CAD build for the part. Positions are in the model's coordinates, mm. A direction names the side the tool comes from. Coordinates: 2 decimals unless noted, no trailing zeros. Loops run counter-clockwise (first coordinate to the right, second up) from the corner with the lowest first, then second, coordinate; pieces in that order, holes last. Notation, with made-up numbers: (-4, 8) - (36, 8) arc R24 ccw to (36, 28) - close; hole circle Ø8 at (-11.75, 44). An arc over 180 degrees is marked (long way). Put each result on its own line as item: value.
```python
from build123d import *

# Parameters (mm, degrees)
SKETCH_1_W          = 15
SKETCH_1_H          = 15
SKETCH_1_W_2        = 13
SKETCH_1_H_2        = 13
EXTRUDE_1_DEPTH     = 460
SKETCH_2_R          = 1.45
CUT_EXTRUDE_1_DEPTH = 461.305605006
SKETCH_3_R          = 1.45
CUT_EXTRUDE_2_DEPTH = 461.305605006


with BuildPart() as part:
    # 草图1 → 拉伸-薄壁1 (new body)
    with BuildSketch(Plane(origin=(0, 0, 0), x_dir=(1, 0, 0), z_dir=(0, 1, 0))):
        Rectangle(SKETCH_1_W, SKETCH_1_H)
        Rectangle(SKETCH_1_W_2, SKETCH_1_H_2, mode=Mode.SUBTRACT)
    extrude(amount=EXTRUDE_1_DEPTH)

    # 草图2 → 切除-拉伸1 (cut, through all)
    with BuildSketch(Plane.XY.offset(7.5)):
        with Locations((0, 7.5)):
            Circle(SKETCH_2_R)
        with Locations((0, 27.5)):
            Circle(SKETCH_2_R)
        with Locations(Location((0, 432.5, 0), (0, 0, 180))):
            Circle(SKETCH_2_R)
        with Locations(Location((0, 452.5, 0), (0, 0, 180))):
            Circle(SKETCH_2_R)
        with Locations((0, 140)):
            Circle(SKETCH_2_R)
        with Locations((0, 160)):
            Circle(SKETCH_2_R)
        with Locations((0, 120)):
            Circle(SKETCH_2_R)
        with Locations(Location((0, 340, 0), (0, 0, 180))):
            Circle(SKETCH_2_R)
        with Locations(Location((0, 300, 0), (0, 0, 180))):
            Circle(SKETCH_2_R)
        with Locations(Location((0, 320, 0), (0, 0, 180))):
            Circle(SKETCH_2_R)
        with Locations((0, 230)):
            Circle(SKETCH_2_R)
        with Locations((0, 255)):
            Circle(SKETCH_2_R)
        with Locations((0, 205)):
            Circle(SKETCH_2_R)
        with Locations((0, 47.5)):
            Circle(SKETCH_2_R)
        with Locations((0, 67.5)):
            Circle(SKETCH_2_R)
        with Locations((0, 87.5)):
            Circle(SKETCH_2_R)
        with Locations((0, 360)):
            Circle(SKETCH_2_R)
        with Locations((0, 380)):
            Circle(SKETCH_2_R)
        with Locations((0, 400)):
            Circle(SKETCH_2_R)
    extrude(amount=-CUT_EXTRUDE_1_DEPTH, mode=Mode.SUBTRACT)

    # 草图3 → 切除-拉伸2 (cut, through all)
    with BuildSketch(Plane(origin=(7.5, 0, 0), x_dir=(0, 0, -1), z_dir=(1, 0, 0))):
        with Locations((0, 152.5)):
            Circle(SKETCH_3_R)
        with Locations((0, 172.5)):
            Circle(SKETCH_3_R)
        with Locations((0, 287.5)):
            Circle(SKETCH_3_R)
        with Locations((0, 307.5)):
            Circle(SKETCH_3_R)
        with Locations((0, 192.5)):
            Circle(SKETCH_3_R)
        with Locations((0, 267.5)):
            Circle(SKETCH_3_R)
    extrude(amount=-CUT_EXTRUDE_2_DEPTH, mode=Mode.SUBTRACT)


solid = part.part
```
Q1. Slice it at B-B, the plane y = 59.5. Give the cut face in (x, z), then the cut area to 3 significant figures.
Determined:
outline: (-7.5, -7.5) - (7.5, -7.5) - (7.5, 7.5) - (-7.5, 7.5) - close; hole (-6.5, -6.5) - (6.5, -6.5) - (6.5, 6.5) - (-6.5, 6.5) - close
area: 56.0 mm2
Q2. Slice it at A-A, the plane x = 4.25. Give the cut face in (y, z).
Determined:
outline: (0, -7.5) - (460, -7.5) - (460, -6.5) - (0, -6.5) - close; (0, 6.5) - (460, 6.5) - (460, 7.5) - (0, 7.5) - close
Q3. Mould opens along Z. For faces 1 (the flat face through (0, 227, -7.5)), 2 (the flat face through (-7.5, 227, 0)), 3 (the flat face through (6.5, 227, 0)) say: +Z half, -Z half, draft (parallel to the pull), parting line (faces both ways), or undercut.
Determined:
face 1: -Z half
face 2: draft
face 3: undercut
Q4. Tool access for faces 4 (the flat face through (0, 227, 7.5)), 5 (the flat face through (0, 227, -6.5)): list every direction of +Z, -Z, +X, -X, +Y, -Y with a clear straight run to the whole face (end or side of a thin tool).
Determined:
face 4: +Z, +X, -X, +Y, -Y
face 5: +Y, -Y
Q5. Wall check: L1, parallel to Z at x = 2, y = 333; L2, parallel to Z at x = 6.8, y = 192.5. Give the ranges that are in metal, low to high. Write a range as from..to.
Determined:
L1: -7.5..-6.5, 6.5..7.5
L2: -7.5..-1.45, 1.45..7.5
Q6. Pin check, flat tip, straight feed: pin 1 Ø3.5 at (x, y) = (0, 67.5) entering from -Z. Stop position of the tip, or through.
Determined:
pin 1: z = -7.5
